Input: part model. Units: mm. Frame: model coordinates. Face numbers are marked on the shaded views. A direction names the side the tool comes from. Coordinates: 2 decimals unless noted, no trailing zeros. Loops run counter-clockwise (first coordinate to the right, second up) from the corner with the lowest first, then second, coordinate; pieces in that order, holes last. Notation, with made-up numbers: (89, -35) - (128, -35) arc R26 ccw to (128, -20) - close; hole circle Ø4 at (29.5, 65). An arc over 180 degrees is marked (long way). Use a Markdown table: item, result. Add a question column.
1. Access query for the marked faces 1 and 2. Directions: +Z, -Z, +X, -X, +Y, -Y. A direction counts if a zero-diameter tool reaches every point of the face in a straight line with its end or side. Return the directions, or none.
2. Section query A-A on y = 0. Return the cut outline in (x, z), then the cut area to 3 significant figures.
3. Ray query, L1, parallel to X at y = 3.5, z = -1.5; L2, parallel to Y at x = 29.5, z = 0; L3, parallel to X at y = -1, z = -3.25. Return the intervals inside material, ascending. Write a range as [from, to].
4. Contact query for flat-ended pins moving along their axis: P1, Ø2, axis at y = 3.5, z = -3, coming from the +X side; P2, Ø4, axis at x = 16, y = 0.5, coming from the -Z side; P3, Ø1.5, axis at x = 12, z = 0, coming from the +Y side. Output: stop coordinate, or through.
5. Section query B-B on x = 1. Return the cut outline in (y, z), then the cut area to 3 significant figures.
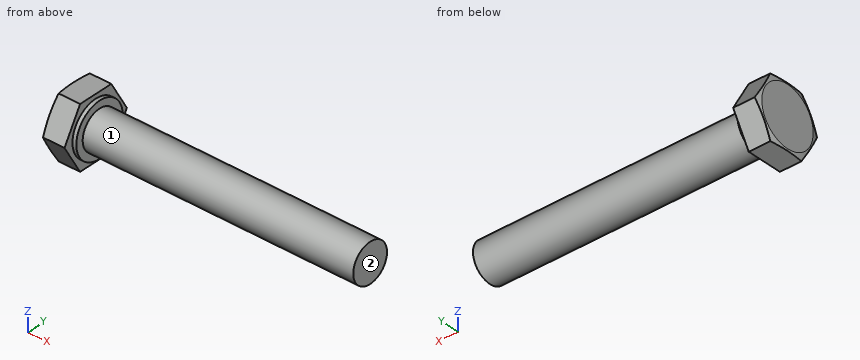
```python
from build123d import *

# Parameters (mm, degrees)
HEAD_DEPTH        = 3.5
SK2_W             = 0.5
SK2_H             = 1.178802154
SK3_R             = 2.5
BODY_DEPTH        = 35
SK5_OUTSIDE_W     = 316.508
SK5_OUTSIDE_H     = 317.746
SK5_OUTSIDE_R     = 3.8
HEADCHAMFER_DEPTH = 39.981833376
HEADCHAMFER_DRAFT = -75


with BuildPart() as part:
    # Sk1 → Head (new body)
    with BuildSketch(Plane(origin=(0, 0, 0), x_dir=(0, 0, -1), z_dir=(1, 0, 0))):
        Polygon((0, 4.618802154), (-4, 2.309401077), (-4, -2.309401077), (0, -4.618802154), (4, -2.309401077), (4, 2.309401077), align=None)
    extrude(amount=-HEAD_DEPTH)

    # Sk2 → UNHead (revolve, cut)
    with BuildSketch(Plane.XY, mode=Mode.PRIVATE) as unhead_sk:
        with Locations((-0.25, 4.029401077)):
            Rectangle(SK2_W, SK2_H)
    revolve(unhead_sk.sketch.rotate(Axis((0, 0, 0), (-1, 0, 0)), 90), axis=Axis((0, 0, 0), (-1, 0, 0)), mode=Mode.SUBTRACT)

    # Sk3 → Body (add)
    with BuildSketch(Plane(origin=(0, 0, 0), x_dir=(0, 0, -1), z_dir=(1, 0, 0))):
        Circle(SK3_R)
    extrude(amount=BODY_DEPTH)


with BuildPart() as headchamfer_tool:
    # Sk5 outside → HeadChamfer (with draft: the straight prism first)
    with BuildSketch(Plane.ZY.offset(3.5)):
        Rectangle(SK5_OUTSIDE_W, SK5_OUTSIDE_H)
        Circle(SK5_OUTSIDE_R, mode=Mode.SUBTRACT)
    extrude(amount=-HEADCHAMFER_DEPTH)
    # HeadChamfer: the draft: its side faces are tilted about the plane it starts from
    headchamfer_sides = [headchamfer_tool.faces().sort_by_distance(p)[0] for p in [
        (16.490916688, -158.873, 0),
        (16.490916688, 0, 158.254),
        (16.490916688, 158.873, 0),
        (16.490916688, 0, -158.254),
        (16.490916688, 0, -3.8),
    ]]
    draft(headchamfer_sides, Plane.ZY.offset(3.5), HEADCHAMFER_DRAFT)


with BuildPart() as part_1:
    add(part.part)

    # HeadChamfer: cut by headchamfer_tool
    add(headchamfer_tool.part, mode=Mode.SUBTRACT)


solid = part_1.part
```
Resolved:
| question | item | result |
|---|---|---|
| 1 | face 1 | +X |
| 1 | face 2 | +Z, -Z, +X, +Y, -Y |
| 2 | outline | (-3.5, -3.8) - (-3.45, -4) - (-0.5, -4) - (-0.5, -3.44) - (0, -3.44) - (0, -2.5) - (35, -2.5) - (35, 2.5) - (0, 2.5) - (0, 3.44) - (-0.5, 3.44) - (-0.5, 4) - (-3.45, 4) - (-3.5, 3.8) - close |
| 2 | area | 202 mm² |
| 3 | L1 | [-3.5, -0.5] |
| 3 | L2 | [-2.5, 2.5] |
| 3 | L3 | [-3.5, 0] |
| 4 | P1 | x = -0.5 |
| 4 | P2 | z = -2.5 |
| 4 | P3 | y = 2.5 |
| 5 | outline | circle Ø5 at (0, 0) |
| 5 | area | 19.6 mm² |
